```python
from build123d import *

# Parameters (mm, degrees)
SKETCH1_R           = 4.826
BOSS_EXTRUDE1_DEPTH = 47.625
SKETCH2_W           = 1.016
SKETCH2_H           = 1.016
FILLET1_R           = 0.254


with BuildPart() as part:
    # Sketch1 → Boss-Extrude1 (new, symmetric)
    with BuildSketch(Plane.XY):
        Circle(SKETCH1_R)
    extrude(amount=BOSS_EXTRUDE1_DEPTH, both=True)

    # Sketch2 → Cut-Revolve1 (revolve, cut)
    with BuildSketch(Plane(origin=(0, 0, 0), x_dir=(1, 0, 0), z_dir=(0, 1, 0))):
        with Locations((-4.318, 43.942)):
            Rectangle(SKETCH2_W, SKETCH2_H)
    revolve(axis=Axis((0, 0, -52.012367131), (0, 0, 1)), mode=Mode.SUBTRACT)

    # Fillet1
    fillet1_edges = [part.edges().sort_by_distance(p)[0] for p in [
        (-4.826, 0, -47.625),
        (-4.826, 0, 47.625),
    ]]
    fillet(fillet1_edges, radius=FILLET1_R)


solid = part.part
```
Geometry: final body of the model. Coordinates: model frame, mm. A direction names the side the tool comes from. Round coordinates to 2 decimals unless told otherwise and drop trailing zeros. Write each loop counter-clockwise with the first axis right and the second up, starting at its lowest first coordinate (ties: lowest second). Pieces come first, ordered by that corner, then holes. Notation, with made-up numbers: M -35,40 L -22,40 A25 cw -22,66 Z; hole C 0,-38.75 d1. An arc over 180 degrees is marked long. Answer in a Markdown table with one row per item. Add a question column.
(1) Reachability of faces 5 (the face through (-3.83, -2.937, -45.89)), 6 (the face through (-4, -1, -43.434)) from +Z, -Z, +X, -X, +Y, -Y: full face, straight path, thin tool, end or side. Return the list, or none.
(2) Contact query for flat-ended pins moving along their axis: pin 1 (1.5 mm diameter, centred on y = -2.5, z = 8.5, fed in from +X); pin 2 (1 mm diameter, centred on y = -2, z = -36.5, fed in from +X); pin 3 (2 mm diameter, centred on x = -1.5, z = 2, fed in from -Y). Output: stop coordinate, or through.
(3) Draft query along Z for faces 1 (the face through (0, 0, 47.625)), 2 (the face through (3.02, 2.32, -43.95)), 3 (the face through (-4, -1, -44.45)), 4 (the face through (-3.83, -2.937, 2.604)). Return one class per face: pulls with the +Z half, pulls with the -Z half, needs draft (parallel to the pull), parting line crosses it, or undercut.
(4) Cut plane A-A, the plane z = 41. Return the cut outline in (x, y), then the cut area to 3 significant figures.
(5) Ray query, L1, parallel to Z at x = 2.75, y = 2.75 (3 decimals); L2, parallel to Y at x = 0.25, z = 21.5; L3, parallel to Z at x = -3.5, y = -3.25. Return the intervals inside material, ascending.
Established:
| question | item | result |
|---|---|---|
| 1 | face 5 | +Z, -Z |
| 1 | face 6 | none |
| 2 | pin 1 | x = 4.5 |
| 2 | pin 2 | x = 4.59 |
| 2 | pin 3 | y = -4.8 |
| 3 | face 1 | pulls with the +Z half |
| 3 | face 2 | undercut |
| 3 | face 3 | undercut |
| 3 | face 4 | needs draft |
| 4 | outline | C 0,0 d9.65 |
| 4 | area | 73.2 mm² |
| 5 | L1 | -47.625 to -44.45, -43.434 to 47.625 |
| 5 | L2 | -4.82 to 4.82 |
| 5 | L3 | -47.52 to -44.45, -43.43 to 47.52 |
